```python
from build123d import *

# Parameters (mm, degrees)
CYLINDER072_R          = 1.6
CYLINDER072_DEPTH      = 10
CYLINDER071_R          = 1.6
CYLINDER071_DEPTH      = 10
CYLINDER070_R          = 1.6
CYLINDER070_DEPTH      = 10
CYLINDER069_R          = 1.6
CYLINDER069_DEPTH      = 10
CYLINDER066_R          = 12
CYLINDER066_DEPTH      = 10
BOX045_W               = 12
BOX045_H               = 12
BOX045_DEPTH           = 4
CUT015_PLACEMENT_ANGLE = 90
CYLINDER067_R          = 12
CYLINDER067_DEPTH      = 10
BOX046_W               = 12
BOX046_H               = 12
BOX046_DEPTH           = 4
CUT016_PLACEMENT_ANGLE = 180
CYLINDER068_R          = 12
CYLINDER068_DEPTH      = 10
BOX047_W               = 12
BOX047_H               = 12
BOX047_DEPTH           = 4
CUT017_PLACEMENT_ANGLE = 270
CYLINDER_R             = 12
CYLINDER_DEPTH         = 10
BOX044_W               = 12
BOX044_H               = 12
BOX044_DEPTH           = 4
CYLINDER063_R          = 1.6
CYLINDER063_DEPTH      = 10
CYLINDER064_R          = 1.6
CYLINDER064_DEPTH      = 10
CYLINDER065_R          = 1.6
CYLINDER065_DEPTH      = 10
CYLINDER062_R          = 1.6
CYLINDER062_DEPTH      = 10
CYLINDER051_R          = 1.6
CYLINDER051_DEPTH      = 10
CYLINDER052_R          = 1.6
CYLINDER052_DEPTH      = 10
CYLINDER050_R          = 1.6
CYLINDER050_DEPTH      = 10
CYLINDER054_R          = 1.6
CYLINDER054_DEPTH      = 20
CYLINDER053_R          = 1.6
CYLINDER053_DEPTH      = 20
CYLINDER056_R          = 1.6
CYLINDER056_DEPTH      = 10
CYLINDER057_R          = 1.6
CYLINDER057_DEPTH      = 10
CYLINDER058_R          = 1.6
CYLINDER058_DEPTH      = 10
CYLINDER059_R          = 1.6
CYLINDER059_DEPTH      = 10
CYLINDER055_R          = 1.6
CYLINDER055_DEPTH      = 10
CYLINDER061_R          = 1.6
CYLINDER061_DEPTH      = 20
CYLINDER060_R          = 1.6
CYLINDER060_DEPTH      = 20
CYLINDER048_R          = 1.6
CYLINDER048_DEPTH      = 10
CYLINDER049_R          = 1.6
CYLINDER049_DEPTH      = 10
CYLINDER047_R          = 1.6
CYLINDER047_DEPTH      = 10
BOX_W                  = 140
BOX_H                  = 113
BOX_DEPTH              = 4


with BuildPart() as cylinder074:
    # Cylinder072 → Cylinder072 (new body)
    with BuildSketch(Plane(origin=(120, 93, 0), x_dir=(1, 0, 0), z_dir=(0, 0, 1))):
        Circle(CYLINDER072_R)
    extrude(amount=CYLINDER072_DEPTH)


with BuildPart() as wallmounts:
    # Cylinder071 → Cylinder071 (new body)
    with BuildSketch(Plane(origin=(20, 93, 0), x_dir=(1, 0, 0), z_dir=(0, 0, 1))):
        Circle(CYLINDER071_R)
    extrude(amount=CYLINDER071_DEPTH)

    # Fusion039: union Cylinder074
    add(cylinder074.part)


with BuildPart() as cylinder072:
    # Cylinder070 → Cylinder070 (new body)
    with BuildSketch(Plane(origin=(125, 71.5, 0), x_dir=(1, 0, 0), z_dir=(0, 0, 1))):
        Circle(CYLINDER070_R)
    extrude(amount=CYLINDER070_DEPTH)


with BuildPart() as cuts001:
    # Cylinder069 → Cylinder069 (new body)
    with BuildSketch(Plane(origin=(15, 71.5, 0), x_dir=(1, 0, 0), z_dir=(0, 0, 1))):
        Circle(CYLINDER069_R)
    extrude(amount=CYLINDER069_DEPTH)

    # Fusion038: union Cylinder072
    add(cylinder072.part)


with BuildPart() as cylinder068:
    # Cylinder066 → Cylinder066 (new body)
    with BuildSketch(Plane(origin=(12, 12, 0), x_dir=(1, 0, 0), z_dir=(0, 0, 1))):
        Circle(CYLINDER066_R)
    extrude(amount=CYLINDER066_DEPTH)


with BuildPart() as cutout001:
    # Box045 → Box045 (new body)
    with BuildSketch(Plane.XY):
        with Locations((6, 6)):
            Rectangle(BOX045_W, BOX045_H)
    extrude(amount=BOX045_DEPTH)

    # Cut015: cut Cylinder068
    add(cylinder068.part, mode=Mode.SUBTRACT)


with BuildPart() as cutout001_1:
    # Cut015 placement: moved
    add(cutout001.part.moved(Location((140, 0, 0))).rotate(Axis((140, 0, 0), (0, 0, 1)), CUT015_PLACEMENT_ANGLE))


with BuildPart() as cylinder069:
    # Cylinder067 → Cylinder067 (new body)
    with BuildSketch(Plane(origin=(12, 12, 0), x_dir=(1, 0, 0), z_dir=(0, 0, 1))):
        Circle(CYLINDER067_R)
    extrude(amount=CYLINDER067_DEPTH)


with BuildPart() as cutout002:
    # Box046 → Box046 (new body)
    with BuildSketch(Plane.XY):
        with Locations((6, 6)):
            Rectangle(BOX046_W, BOX046_H)
    extrude(amount=BOX046_DEPTH)

    # Cut016: cut Cylinder069
    add(cylinder069.part, mode=Mode.SUBTRACT)


with BuildPart() as cutout002_1:
    # Cut016 placement: moved
    add(cutout002.part.moved(Location((140, 113, 0))).rotate(Axis((140, 113, 0), (0, 0, 1)), CUT016_PLACEMENT_ANGLE))


with BuildPart() as cylinder070:
    # Cylinder068 → Cylinder068 (new body)
    with BuildSketch(Plane(origin=(12, 12, 0), x_dir=(1, 0, 0), z_dir=(0, 0, 1))):
        Circle(CYLINDER068_R)
    extrude(amount=CYLINDER068_DEPTH)


with BuildPart() as cutout003:
    # Box047 → Box047 (new body)
    with BuildSketch(Plane.XY):
        with Locations((6, 6)):
            Rectangle(BOX047_W, BOX047_H)
    extrude(amount=BOX047_DEPTH)

    # Cut017: cut Cylinder070
    add(cylinder070.part, mode=Mode.SUBTRACT)


with BuildPart() as cutout003_1:
    # Cut017 placement: moved
    add(cutout003.part.moved(Location((0, 113, 0))).rotate(Axis((0, 113, 0), (0, 0, 1)), CUT017_PLACEMENT_ANGLE))


with BuildPart() as cylinder067:
    # Cylinder → Cylinder (new body)
    with BuildSketch(Plane(origin=(12, 12, 0), x_dir=(1, 0, 0), z_dir=(0, 0, 1))):
        Circle(CYLINDER_R)
    extrude(amount=CYLINDER_DEPTH)


with BuildPart() as cutout004:
    # Box044 → Box044 (new body)
    with BuildSketch(Plane.XY):
        with Locations((6, 6)):
            Rectangle(BOX044_W, BOX044_H)
    extrude(amount=BOX044_DEPTH)

    # Cut014: cut Cylinder067
    add(cylinder067.part, mode=Mode.SUBTRACT)

    # Fusion037: union cutOut001, cutOut002, cutOut003
    add(cutout001_1.part)
    add(cutout002_1.part)
    add(cutout003_1.part)


with BuildPart() as cylinder064:
    # Cylinder063 → Cylinder063 (new body)
    with BuildSketch(Plane(origin=(128, 12, 0), x_dir=(1, 0, 0), z_dir=(0, 0, 1))):
        Circle(CYLINDER063_R)
    extrude(amount=CYLINDER063_DEPTH)


with BuildPart() as cylinder065:
    # Cylinder064 → Cylinder064 (new body)
    with BuildSketch(Plane(origin=(12, 101, 0), x_dir=(1, 0, 0), z_dir=(0, 0, 1))):
        Circle(CYLINDER064_R)
    extrude(amount=CYLINDER064_DEPTH)


with BuildPart() as cylinder066:
    # Cylinder065 → Cylinder065 (new body)
    with BuildSketch(Plane(origin=(128, 101, 0), x_dir=(1, 0, 0), z_dir=(0, 0, 1))):
        Circle(CYLINDER065_R)
    extrude(amount=CYLINDER065_DEPTH)


with BuildPart() as outercuts:
    # Cylinder062 → Cylinder062 (new body)
    with BuildSketch(Plane(origin=(12, 12, 0), x_dir=(1, 0, 0), z_dir=(0, 0, 1))):
        Circle(CYLINDER062_R)
    extrude(amount=CYLINDER062_DEPTH)

    # Fusion036: union Cylinder064, Cylinder065, Cylinder066
    add(cylinder064.part)
    add(cylinder065.part)
    add(cylinder066.part)


with BuildPart() as cylinder052:
    # Cylinder051 → Cylinder051 (new body)
    with BuildSketch(Plane(origin=(27.25, 23, 0), x_dir=(1, 0, 0), z_dir=(0, 0, 1))):
        Circle(CYLINDER051_R)
    extrude(amount=CYLINDER051_DEPTH)


with BuildPart() as cylinder053:
    # Cylinder052 → Cylinder052 (new body)
    with BuildSketch(Plane(origin=(17.25, 53, 0), x_dir=(1, 0, 0), z_dir=(0, 0, 1))):
        Circle(CYLINDER052_R)
    extrude(amount=CYLINDER052_DEPTH)


with BuildPart() as obj1:
    # Cylinder050 → Cylinder050 (new body)
    with BuildSketch(Plane(origin=(7.25, 23, 0), x_dir=(1, 0, 0), z_dir=(0, 0, 1))):
        Circle(CYLINDER050_R)
    extrude(amount=CYLINDER050_DEPTH)

    # Fusion031: union Cylinder052, Cylinder053
    add(cylinder052.part)
    add(cylinder053.part)


with BuildPart() as obj1_1:
    # Fusion031 placement: moved
    add(obj1.part.moved(Location((105.8, 0, 0))))


with BuildPart() as cylinder055:
    # Cylinder054 → Cylinder054 (new body)
    with BuildSketch(Plane(origin=(44.35, 40.35, 0), x_dir=(1, 0, 0), z_dir=(0, 0, 1))):
        Circle(CYLINDER054_R)
    extrude(amount=CYLINDER054_DEPTH)


with BuildPart() as obj2:
    # Cylinder053 → Cylinder053 (new body)
    with BuildSketch(Plane(origin=(2.75, 2.75, 0), x_dir=(1, 0, 0), z_dir=(0, 0, 1))):
        Circle(CYLINDER053_R)
    extrude(amount=CYLINDER053_DEPTH)

    # Fusion032: union Cylinder055
    add(cylinder055.part)


with BuildPart() as obj2_1:
    # Fusion032 placement: moved
    add(obj2.part.moved(Location((46.5, 13, 0))))


with BuildPart() as cylinder057:
    # Cylinder056 → Cylinder056 (new body)
    with BuildSketch(Plane(origin=(90, 65, 0), x_dir=(1, 0, 0), z_dir=(0, 0, 1))):
        Circle(CYLINDER056_R)
    extrude(amount=CYLINDER056_DEPTH)


with BuildPart() as cylinder058:
    # Cylinder057 → Cylinder057 (new body)
    with BuildSketch(Plane(origin=(100, 95, 0), x_dir=(1, 0, 0), z_dir=(0, 0, 1))):
        Circle(CYLINDER057_R)
    extrude(amount=CYLINDER057_DEPTH)


with BuildPart() as cylinder059:
    # Cylinder058 → Cylinder058 (new body)
    with BuildSketch(Plane(origin=(40, 95, 0), x_dir=(1, 0, 0), z_dir=(0, 0, 1))):
        Circle(CYLINDER058_R)
    extrude(amount=CYLINDER058_DEPTH)


with BuildPart() as cylinder060:
    # Cylinder059 → Cylinder059 (new body)
    with BuildSketch(Plane(origin=(70, 105, 0), x_dir=(1, 0, 0), z_dir=(0, 0, 1))):
        Circle(CYLINDER059_R)
    extrude(amount=CYLINDER059_DEPTH)


with BuildPart() as obj3:
    # Cylinder055 → Cylinder055 (new body)
    with BuildSketch(Plane(origin=(50, 65, 0), x_dir=(1, 0, 0), z_dir=(0, 0, 1))):
        Circle(CYLINDER055_R)
    extrude(amount=CYLINDER055_DEPTH)

    # Fusion033: union Cylinder057, Cylinder058, Cylinder059, Cylinder060
    add(cylinder057.part)
    add(cylinder058.part)
    add(cylinder059.part)
    add(cylinder060.part)


with BuildPart() as cylinder062:
    # Cylinder061 → Cylinder061 (new body)
    with BuildSketch(Plane(origin=(100.5, 41, 0), x_dir=(1, 0, 0), z_dir=(0, 0, 1))):
        Circle(CYLINDER061_R)
    extrude(amount=CYLINDER061_DEPTH)


with BuildPart() as obj4:
    # Cylinder060 → Cylinder060 (new body)
    with BuildSketch(Plane(origin=(39.5, 41, 0), x_dir=(1, 0, 0), z_dir=(0, 0, 1))):
        Circle(CYLINDER060_R)
    extrude(amount=CYLINDER060_DEPTH)

    # Fusion034: union Cylinder062
    add(cylinder062.part)


with BuildPart() as cylinder049:
    # Cylinder048 → Cylinder048 (new body)
    with BuildSketch(Plane(origin=(27.25, 23, 0), x_dir=(1, 0, 0), z_dir=(0, 0, 1))):
        Circle(CYLINDER048_R)
    extrude(amount=CYLINDER048_DEPTH)


with BuildPart() as cylinder050:
    # Cylinder049 → Cylinder049 (new body)
    with BuildSketch(Plane(origin=(17.25, 53, 0), x_dir=(1, 0, 0), z_dir=(0, 0, 1))):
        Circle(CYLINDER049_R)
    extrude(amount=CYLINDER049_DEPTH)


with BuildPart() as cuts:
    # Cylinder047 → Cylinder047 (new body)
    with BuildSketch(Plane(origin=(7.25, 23, 0), x_dir=(1, 0, 0), z_dir=(0, 0, 1))):
        Circle(CYLINDER047_R)
    extrude(amount=CYLINDER047_DEPTH)

    # Fusion: union Cylinder049, Cylinder050
    add(cylinder049.part)
    add(cylinder050.part)

    # Fusion035: union obj1, obj2, obj3, obj4
    add(obj1_1.part)
    add(obj2_1.part)
    add(obj3.part)
    add(obj4.part)


with BuildPart() as base008:
    # Box → Box (new body)
    with BuildSketch(Plane.XY):
        with Locations((70, 56.5)):
            Rectangle(BOX_W, BOX_H)
    extrude(amount=BOX_DEPTH)

    # Cut: cut cuts
    add(cuts.part, mode=Mode.SUBTRACT)

    # Cut013: cut outerCuts
    add(outercuts.part, mode=Mode.SUBTRACT)

    # Cut018: cut cutOut004
    add(cutout004.part, mode=Mode.SUBTRACT)

    # Cut019: cut cuts001
    add(cuts001.part, mode=Mode.SUBTRACT)

    # Cut020: cut wallMounts
    add(wallmounts.part, mode=Mode.SUBTRACT)


solid = base008.part
```
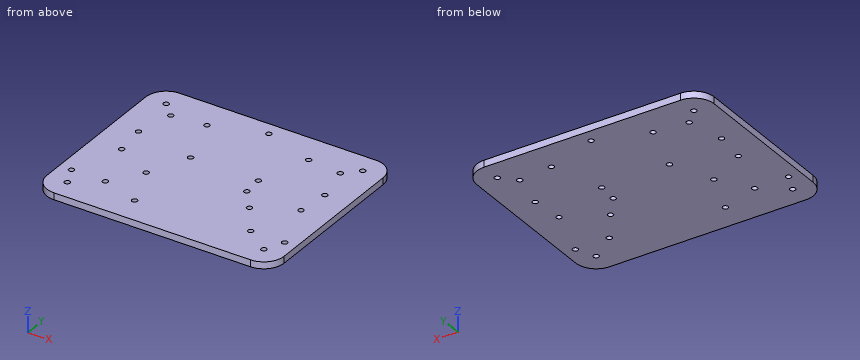
Verification items for the finished model (mm, model axes). Coordinates: 2 decimals unless noted, no trailing zeros. Loops run counter-clockwise (first coordinate to the right, second up) from the corner with the lowest first, then second, coordinate; pieces in that order, holes last. Notation, with made-up numbers: (17, -8) -> (51, -8) arc R20 cw to (51, 18) -> close; hole circle Ø1 at (10, -13.5). An arc over 180 degrees is marked (long way). Answer in a Markdown table with one row per item.
1) Depth check by flat-ended pin: P1, Ø1.9, axis at x = 100, y = 95, coming from the +Z side. Enter the tip coordinate at first touch or a pass-through.
The answers:
| item | result |
|---|---|
| P1 | passes through |
2) Section check A-A (x = 120). Record the cut outline in (y, z), and give its area (3 significant figures).
The answers:
| item | result |
|---|---|
| outline | (0, 0) -> (91.4, 0) -> (91.4, 4) -> (0, 4) -> close; (94.6, 0) -> (113, 0) -> (113, 4) -> (94.6, 4) -> close |
| area | 439 mm2 |
3) Section check B-B (y = 71.5). Record the cut outline in (x, z).
The answers:
| item | result |
|---|---|
| outline | (0, 0) -> (13.4, 0) -> (13.4, 4) -> (0, 4) -> close; (16.6, 0) -> (123.4, 0) -> (123.4, 4) -> (16.6, 4) -> close; (126.6, 0) -> (140, 0) -> (140, 4) -> (126.6, 4) -> close |
4) Section check D-D (z = 2.1). Give the number of separate pieces and of enclosed holes in the cut face, and give its area (3 significant figures).
The answers:
| item | result |
|---|---|
| separate pieces | 1 |
| enclosed holes | 23 |
| area | 15,500 mm2 |
5) Section check C-C (y = 23). Record the cut outline in (x, z).
The answers:
| item | result |
|---|---|
| outline | (0, 0) -> (5.65, 0) -> (5.65, 4) -> (0, 4) -> close; (8.85, 0) -> (25.65, 0) -> (25.65, 4) -> (8.85, 4) -> close; (28.85, 0) -> (111.45, 0) -> (111.45, 4) -> (28.85, 4) -> close; (114.65, 0) -> (131.45, 0) -> (131.45, 4) -> (114.65, 4) -> close; (134.65, 0) -> (140, 0) -> (140, 4) -> (134.65, 4) -> close |
6) Scan lines: line 1 along Y through (x, z) = (12, 1.55); line 2 along X through (y, z) = (41, 2.4); line 3 along X through (y, z) = (15.75, 1.5). Record each from-to range of solid material in increasing order. Write a range as from..to.
The answers:
| item | result |
|---|---|
| line 1 | y = 0..10.4, 13.6..99.4, 102.6..113 |
| line 2 | x = 0..37.9, 41.1..98.9, 102.1..140 |
| line 3 | x = 0..47.65, 50.85..140 |
